Verification items for the finished model (mm, model axes). A direction names the side the tool comes from. Round coordinates to 2 decimals unless told otherwise and drop trailing zeros. Order: outer loops, then holes, each group sorted by start corner. A loop starts at its lowest first (then second) coordinate and runs counter-clockwise, first axis right, second up. Notation, with made-up numbers: (0, 50.25) -> (45, 50.25) arc R26 ccw to (45, 72.25) -> close; hole circle Ø3 at (86.25, 42). An arc over 180 degrees is marked (long way). Put each result on its own line as item: value.
from build123d import *

# Parameters (mm, degrees)
BOSS_EXTRUDE1_DEPTH     = 7
SKETCH1_3_W             = 14
SKETCH1_3_H             = 28
SKETCH1_3_W_2           = 7
SKETCH1_3_H_2           = 14
BOSS_EXTRUDE2_DEPTH     = 28
CUT_EXTRUDE1_DEPTH      = 1
CUT_EXTRUDE1_DEPTH_BACK = 28


with BuildPart() as part:
    # Sketch1 → Boss-Extrude1 (new body)
    with BuildSketch(Plane(origin=(0, 0, 0), x_dir=(1, 0, 0), z_dir=(0, 1, 0))):
        Polygon((-15, 0), (0, 0), (0, 14), (14, 14), (14, 28), (-15, 28), align=None)
    extrude(amount=BOSS_EXTRUDE1_DEPTH)

    # Sketch1<3> → Boss-Extrude2 (add)
    with BuildSketch(Plane(origin=(0, 0, 0), x_dir=(1, 0, 0), z_dir=(0, 1, 0))):
        with Locations((-22, 14)):
            Rectangle(SKETCH1_3_W, SKETCH1_3_H)
        with Locations((17.5, 21)):
            Rectangle(SKETCH1_3_W_2, SKETCH1_3_H_2)
    extrude(amount=BOSS_EXTRUDE2_DEPTH)

    # Sketch2 → Cut-Extrude1 (cut, two sides)
    with BuildSketch(Plane.ZY.offset(29)) as cut_extrude1_sk:
        with BuildLine():
            Line((-21, 108), (-21, 28))
            Line((-21, 28), (-21, 21))
            ThreePointArc((-21, 21), (-14, 14), (-7, 21))
            Line((-7, 21), (-7, 28))
            Line((-7, 28), (-7, 108))
            Line((-7, 108), (-7, 268))
            Line((-7, 268), (-21, 268))
            Line((-21, 268), (-21, 108))
        make_face()
    extrude(amount=CUT_EXTRUDE1_DEPTH, mode=Mode.SUBTRACT)
    extrude(cut_extrude1_sk.sketch, amount=-CUT_EXTRUDE1_DEPTH_BACK, mode=Mode.SUBTRACT)


solid = part.part
Item 1: Gauge pin test, flat ends, axial feed: pin 1 Ø10.5 at (x, y) = (6, 18.5) entering from +Z; pin 2 Ø2 at (x, y) = (15, 7) entering from +Z; pin 3 Ø6.5 at (y, z) = (18, -9.5) entering from +X; pin 4 Ø7.5 at (y, z) = (5, -7.5) entering from +X. Record the tip position at first contact, or that the pin passes through.
Check sheet entries:
pin 1: passes through
pin 2: stops at z = -14
pin 3: stops at x = -15
pin 4: stops at x = 0
Item 2: Release check for a two-part mould opening along Z. For faces 6 (the flat face through (-22, 28, -25)), 7 (the flat face through (-22, 25, -21)), 8 (the flat face through (15, 11, -14)) record: +Z half, -Z half, draft (parallel to the pull), parting line (faces both ways), or undercut.
Check sheet entries:
face 6: draft
face 7: undercut
face 8: +Z half
Item 3: Tool access check on faces 1 (the flat face through (-21, 11, 0)), 2 (the flat face through (-22, 24, -7)), 3 (the flat face through (0, 3, -7)), 4 (the flat face through (-4, 7, -17)), 5 (the cylindrical face through (-22, 14, -14)). Record the directions out of +Z, -Z, +X, -X, +Y, -Y that give a thin tool (end or side, any length) a straight path to the whole face; none if there is none.
Check sheet entries:
face 1: +Z, +X, -X, +Y, -Y
face 2: +X, -X, +Y
face 3: +Z, +X, +Y, -Y
face 4: +Z, -Z, +Y
face 5: -X, +Y
Item 4: Section check B-B on x = -25. Record the boundary of the cut face in (y, z).
Check sheet entries:
outline: (0, -28) -> (28, -28) -> (28, -21) -> (21, -21) arc R7 cw to (21, -7) -> (28, -7) -> (28, 0) -> (0, 0) -> close
Item 5: Section check A-A on y = 23. Record the boundary of the cut face in (x, z).
Check sheet entries:
outline: (-29, -28) -> (-15, -28) -> (-15, -21) -> (-29, -21) -> close; (-29, -7) -> (-15, -7) -> (-15, 0) -> (-29, 0) -> close; (14, -28) -> (21, -28) -> (21, -14) -> (14, -14) -> close
Item 6: Material ranges on L1, parallel to X at y = 13.75, z = -23.25; L2, parallel to Y at x = -3, z = -1.25; L3, parallel to X at y = 10, z = -2.5, recorded low to high. Write a range as [from, to].
Check sheet entries:
L1: x = [-29, -15], [14, 21]
L2: y = [0, 7]
L3: x = [-29, -15]
Item 7: Section check D-D on z = -1.75. Record the boundary of the cut face in (x, y).
Check sheet entries:
outline: (-29, 0) -> (0, 0) -> (0, 7) -> (-15, 7) -> (-15, 28) -> (-29, 28) -> close
Item 8: Section check C-C on y = 13. Record the boundary of the cut face in (x, z), then the cut area to 3 significant figures.
Check sheet entries:
outline: (-29, -28) -> (-15, -28) -> (-15, 0) -> (-29, 0) -> close; (14, -28) -> (21, -28) -> (21, -14) -> (14, -14) -> close
area: 490 mm^2
